```python
from build123d import *

# Parameters (mm, degrees)
SKETCH3_W               = 93.7006
SKETCH3_H               = 187.4012
SKETCH3_W_2             = 15.8115
SKETCH3_H_2             = 93.7006
CUT_EXTRUDE1_DEPTH      = 23.0124
HOLE1_D                 = 20.6248
HOLE1_DEPTH             = 27.94
HOLE1_TIP               = 5.953866916
SKETCH7_W               = 10.3124
SKETCH7_H               = 12.7
SKETCH9_R               = 4.7879
CUT_EXTRUDE2_DEPTH      = 11.858625
CUT_EXTRUDE2_DEPTH_BACK = 11.858625


with BuildPart() as part:
    # Sketch1 → Revolve1 (revolve)
    with BuildSketch(Plane.XY):
        Polygon((0, 0), (0, 21.63445), (0.762, 22.39645), (5.8166, 22.39645), (6.8707, 21.34235), (7.9248, 21.34235), (7.9248, 23.42515), (34.1376, 23.42515), (34.8996, 22.66315), (34.8996, 0), align=None)
    revolve(axis=Axis((34.8996, 0, 0), (-1, 0, 0)))

    # Sketch2 → Revolve2 (revolve)
    with BuildSketch(Plane.XY):
        with BuildLine():
            Line((34.8996, 0), (34.8996, 13.08735))
            Line((34.8996, 13.08735), (37.2872, 13.08735))
            Line((37.2872, 13.08735), (37.2872, 12.46505))
            ThreePointArc((37.2872, 12.46505), (37.629416437, 11.638866437), (38.4556, 11.29665))
            Line((38.4556, 11.29665), (40.0685, 11.29665))
            ThreePointArc((40.0685, 11.29665), (40.176691084, 11.301669903), (40.283952505, 11.316686478))
            Line((40.283952505, 11.316686478), (40.894683563, 11.43127))
            Line((40.894683563, 11.43127), (42.163413563, 12.7))
            Line((42.163413563, 12.7), (59.05627, 12.7))
            Line((59.05627, 12.7), (60.325, 11.43127))
            Line((60.325, 11.43127), (60.325, 0))
            Line((60.325, 0), (34.8996, 0))
        make_face()
    revolve(axis=Axis((60.325, 0, 0), (-1, 0, 0)))

    # Sketch3 → Cut-Extrude1 (cut)
    with BuildSketch(Plane(origin=(60.325, 0, 0), x_dir=(0, 0, -1), z_dir=(1, 0, 0))):
        Rectangle(SKETCH3_W, SKETCH3_H)
        Rectangle(SKETCH3_W_2, SKETCH3_H_2, mode=Mode.SUBTRACT)
    extrude(amount=-CUT_EXTRUDE1_DEPTH, mode=Mode.SUBTRACT)

    # Hole1
    with Locations(Plane.ZY):
        with Locations((0, 0)):
            Hole(HOLE1_D / 2, depth=HOLE1_DEPTH)
            with Locations((0, 0, -(HOLE1_DEPTH + HOLE1_TIP / 2))):  # 120° drill point
                Cone(0, HOLE1_D / 2, HOLE1_TIP, mode=Mode.SUBTRACT)

    # Sketch6 → Cut-Revolve1 (revolve, cut)
    with BuildSketch(Plane(origin=(0, 0, 0), x_dir=(1, 0, 0), z_dir=(0, 0.999847695, 0.017452406))):
        Polygon((19.05, 0), (25.187961617, 0), (25.187961617, -14.96695), (25.452022746, -23.42515), (19.05, -23.42515), align=None)
    revolve(axis=Axis((19.05, -0.408825239, 23.421582236), (0, 0.017452406, -0.999847695)), mode=Mode.SUBTRACT)

    # Sketch7 → Cut-Revolve2 (revolve, cut)
    with BuildSketch(Plane.XY):
        with Locations((5.1562, 6.35)):
            Rectangle(SKETCH7_W, SKETCH7_H)
    revolve(axis=Axis((10.3124, 0, 0), (-1, 0, 0)), mode=Mode.SUBTRACT)

    # Sketch8 → Revolve3 (revolve)
    with BuildSketch(Plane.XY):
        with BuildLine():
            Line((6.362790712, 23.340981804), (7.789783697, 21.913988819))
            ThreePointArc((7.789783697, 21.913988819), (7.826981136, 21.824186258), (7.789783697, 21.734383697))
            Line((7.789783697, 21.734383697), (7.39775, 21.34235))
            Line((7.39775, 21.34235), (6.8707, 21.34235))
            Line((6.8707, 21.34235), (6.8707, 21.08835))
            Line((6.8707, 21.08835), (7.9248, 21.08835))
            Line((7.9248, 21.08835), (7.9248, 22.066340712))
            Line((7.9248, 22.066340712), (6.565990712, 23.42515))
            Line((6.565990712, 23.42515), (6.362790712, 23.42515))
            Line((6.362790712, 23.42515), (6.362790712, 23.340981804))
        make_face()
    revolve(axis=Axis((7.9248, 0, 0), (-1, 0, 0)))

    # Sketch9 → Cut-Extrude2 (cut, two sides)
    with BuildSketch(Plane.XY) as cut_extrude2_sk:
        with Locations((47.625, 0)):
            Circle(SKETCH9_R)
    extrude(amount=CUT_EXTRUDE2_DEPTH, mode=Mode.SUBTRACT)
    extrude(cut_extrude2_sk.sketch, amount=-CUT_EXTRUDE2_DEPTH_BACK, mode=Mode.SUBTRACT)


solid = part.part
```
Geometry check sheet. Reference: the model listing, model coordinates, mm. A direction names the side the tool comes from. Coordinates: 2 decimals unless noted, no trailing zeros. Write each loop counter-clockwise with the first axis right and the second up, starting at its lowest first coordinate (ties: lowest second). Pieces come first, ordered by that corner, then holes. Notation, with made-up numbers: (34, 64) -> (87, 64) arc R22 ccw to (87, 88) -> close; hole circle Ø10 at (-34.5, 26.25). An arc over 180 degrees is marked (long way). Use CSV: the item, a comma, the result in double quotes. Start each with the question number.
Item 1: Cross-section at C-C, the plane x = 27. Record the cut outline in (y, z), plus the area to 3 significant figures.
Item 2: Mould release check, pull along X, two halves, no side actions. Record for faces 1 (the cylindrical face through (36.11, -2.837, 12.776)), 2 (the conical face through (60.122, -11.633, -0.124)), 3 (the cylindrical face through (22.35, -5.39, 12.32)), 4 (the cylindrical face through (7.138, -4.627, 20.835)): released by +X, released by -X, zero draft, split by the parting line, or undercut.
Item 3: Cross-section at B-B, the plane x = 9.5. Record the cut outline in (y, z), plus the area to 3 significant figures.
Item 4: Set-up check for faces 5 (the cylindrical face through (52.05, -1.83, 0.11)), 6 (the conical face through (41.115, 11.651, 0.125)), 7 (the flat face through (54, 0, -7.906)), 8 (the cylindrical face through (50.7, -12.7, -0.1)), 9 (the cylindrical face through (50.7, 12.7, 0.1)): record each of +Z, -Z, +X, -X, +Y, -Y from which the full face is reachable in a straight line by a thin tool's end or side.
Item 5: Depth check by flat-ended pin: pin 1 Ø23.5 at (y, z) = (0, 0) entering from -X; pin 2 Ø7.5 at (x, y) = (47.625, 0) entering from +Z; pin 3 Ø12 at (x, z) = (53, -7.5) entering from -Y; pin 4 Ø10 at (x, y) = (46.5, 2.5) entering from +Z. Enter the tip coordinate at first touch or a pass-through.
Item 6: Thickness scan on line 1 (Z direction, x = 2, y = 0); line 2 (X direction, y = 0, z = 0) (3 decimals). Record the ranges inside material, lowest first.
Item 7: Cross-section at A-A, the plane x = 44. Record the cut outline in (y, z).
Answers:
1,outline,"circle Ø46.85 at (0, 0); hole circle Ø20.62 at (0, 0)"
1,area,"1,390 mm^2"
2,face 1,"zero draft"
2,face 2,"released by +X"
2,face 3,"undercut"
2,face 4,"undercut"
3,outline,"circle Ø46.85 at (0, 0); hole circle Ø25.4 at (0, 0)"
3,area,"1,220 mm^2"
4,face 5,"+Z, -Z"
4,face 6,"+Y"
4,face 7,"-Z, +X, +Y, -Y"
4,face 8,"+X, -Y"
4,face 9,"+X, +Y"
5,pin 1,"x = 10.31"
5,pin 2,"through"
5,pin 3,"y = -12.61"
5,pin 4,"z = 7.91"
6,line 1,"-22.4 to -12.7, 12.7 to 22.4"
6,line 2,"33.894 to 42.837, 52.413 to 60.325"
7,outline,"(-9.94, -7.91) -> (-3.13, -7.91) -> (-3.13, 7.91) -> (-9.94, 7.91) arc R12.7 ccw to start; (3.13, -7.91) -> (9.94, -7.91) arc R12.7 ccw to (9.94, 7.91) -> (3.13, 7.91) -> close"
